```python
from build123d import *

# Parameters (mm, degrees)
SKETCH1_W           = 55
SKETCH1_H           = 35
SKETCH1_R           = 9.55
SKETCH1_R_2         = 1.5
BOSS_EXTRUDE3_DEPTH = 6
SKETCH4_W           = 55
SKETCH4_H           = 35
BOSS_EXTRUDE5_DEPTH = 2
SKETCH8_W           = 8.5
SKETCH8_H           = 35
BOSS_EXTRUDE6_DEPTH = 55
SKETCH9_R           = 2
CUT_EXTRUDE1_DEPTH  = 8.5
FILLET1_R           = 2


with BuildPart() as part:
    # Sketch1 → Boss-Extrude3 (new body)
    with BuildSketch(Plane.XY):
        with Locations((27.5, 17.5)):
            Rectangle(SKETCH1_W, SKETCH1_H)
        with Locations((35, 17.5)):
            Circle(SKETCH1_R, mode=Mode.SUBTRACT)
        with Locations((44.192388155, 26.692388155)):
            Circle(SKETCH1_R_2, mode=Mode.SUBTRACT)
        with Locations((44.192388155, 8.307611845)):
            Circle(SKETCH1_R_2, mode=Mode.SUBTRACT)
        with Locations((25.807611845, 8.307611845)):
            Circle(SKETCH1_R_2, mode=Mode.SUBTRACT)
        with Locations((25.807611845, 26.692388155)):
            Circle(SKETCH1_R_2, mode=Mode.SUBTRACT)
    extrude(amount=BOSS_EXTRUDE3_DEPTH)

    # Sketch4 → Boss-Extrude5 (add)
    with BuildSketch(Plane.XY.offset(6)):
        with Locations((27.5, 17.5)):
            Rectangle(SKETCH4_W, SKETCH4_H)
        with BuildLine():
            ThreePointArc((28.799419693, 26.47083501), (23.686291501, 28.813708499), (26.02916499, 23.700580307))
            ThreePointArc((26.02916499, 23.700580307), (26.263454109, 23.57743344), (26.255822455, 23.312861521))
            ThreePointArc((26.255822455, 23.312861521), (24.5, 17.5), (26.255822455, 11.687138479))
            ThreePointArc((26.255822455, 11.687138479), (26.263454109, 11.42256656), (26.02916499, 11.299419693))
            ThreePointArc((26.02916499, 11.299419693), (23.686291501, 6.186291501), (28.799419693, 8.52916499))
            ThreePointArc((28.799419693, 8.52916499), (28.92256656, 8.763454109), (29.187138479, 8.755822455))
            ThreePointArc((29.187138479, 8.755822455), (35, 7), (40.812861521, 8.755822455))
            ThreePointArc((40.812861521, 8.755822455), (41.07743344, 8.763454109), (41.200580307, 8.52916499))
            ThreePointArc((41.200580307, 8.52916499), (46.313708499, 6.186291501), (43.97083501, 11.299419693))
            ThreePointArc((43.97083501, 11.299419693), (43.736545891, 11.42256656), (43.744177545, 11.687138479))
            ThreePointArc((43.744177545, 11.687138479), (45.5, 17.5), (43.744177545, 23.312861521))
            ThreePointArc((43.744177545, 23.312861521), (43.736545891, 23.57743344), (43.97083501, 23.700580307))
            ThreePointArc((43.97083501, 23.700580307), (46.313708499, 28.813708499), (41.200580307, 26.47083501))
            ThreePointArc((41.200580307, 26.47083501), (41.07743344, 26.236545891), (40.812861521, 26.244177545))
            ThreePointArc((40.812861521, 26.244177545), (35, 28), (29.187138479, 26.244177545))
            ThreePointArc((29.187138479, 26.244177545), (28.92256656, 26.236545891), (28.799419693, 26.47083501))
        make_face(mode=Mode.SUBTRACT)
    extrude(amount=BOSS_EXTRUDE5_DEPTH)

    # Sketch8 → Boss-Extrude6 (add)
    with BuildSketch(Plane(origin=(0, 0, 0), x_dir=(-1, 0, 0), z_dir=(0, 0, -1))):
        with Locations((-4.25, 17.5)):
            Rectangle(SKETCH8_W, SKETCH8_H)
    extrude(amount=BOSS_EXTRUDE6_DEPTH)

    # Sketch9 → Cut-Extrude1 (cut)
    with BuildSketch(Plane.ZY):
        with Locations((-47, 27)):
            Circle(SKETCH9_R)
        with Locations((-47, 8)):
            Circle(SKETCH9_R)
        with Locations((-8.5, 27)):
            Circle(SKETCH9_R)
        with Locations((-8.5, 8)):
            Circle(SKETCH9_R)
        with Locations((-23.5, 17.5)):
            Circle(SKETCH9_R)
    extrude(amount=-CUT_EXTRUDE1_DEPTH, mode=Mode.SUBTRACT)

    # Fillet1
    fillet1_edges = [part.edges().sort_by_distance(p)[0] for p in [
        (8.5, 17.5, 0),
    ]]
    fillet(fillet1_edges, radius=FILLET1_R)


solid = part.part
```
Part model, mm, in its own coordinate system. A direction names the side the tool comes from. Coordinates: 2 decimals unless noted, no trailing zeros. Order: outer loops, then holes, each group sorted by start corner. A loop starts at its lowest first (then second) coordinate and runs counter-clockwise, first axis right, second up. Notation, with made-up numbers: (76.25, 72.5) - (102.25, 72.5) arc R23 cw to (102.25, 88.5) - close; hole circle Ø2 at (57, 65.5). An arc over 180 degrees is marked (long way). Return JSON: item names as keys, results as strings. Group by question number.
Item 1: Cut at C-C (x = 6.5). List the corners of the cut face in (y, z), plus the area to 3 significant figures.
Item 2: Cut at D-D (z = -40.5). List the corners of the cut face in (x, y), plus the area to 4 significant figures.
Item 3: Cut at A-A (x = 35). List the corners of the cut face in (y, z), plus the area to 3 significant figures.
Item 4: Which spindle directions (+Z, -Z, +X, -X, +Y, -Y) get a long thin tool onto all of the face, cutting with end or side? Do faces 4 (the face through (4.19, 19.483, -23.76)), 5 (the face through (27.5, 25.5, 0)), 6 (the face through (45.5, 17.4, 7)). Say none if no direction does.
Item 5: Pull direction Z, two halves, no side cores. Call faces 1 (the face through (7, 35, -14)), 2 (the face through (4.19, 9.352, -9.974)), 3 (the face through (39, 27, 6)): pulls with the +Z half, pulls with the -Z half, needs draft (parallel to the pull), parting line crosses it, or undercut.
Item 6: Cut at B-B (z = -23.5). List the corners of the cut face in (x, y).
Item 7: Pin check, flat tips, straight feed: pin 1 (2.5 mm diameter, centred on x = 44.19, y = 8.31, fed in from -Z); pin 2 (5.5 mm diameter, centred on x = 44.19, y = 26.69, fed in from -Z); pin 3 (5 mm diameter, centred on y = 31, z = -42.5, fed in from +X); pin 4 (3.5 mm diameter, centred on x = 25.81, y = 26.69, fed in from +Z). Stop position of each tip, or through.
Item 8: Drill centre lines: probe 1 along Y at (x, z) = (3, -47); probe 2 along Y at (x, z) = (3.5, -23.5); probe 3 along Y at (x, z) = (26.5, 2.5). Where is each one in solid material? Low to high. Write a range as from..to.
Check values:
{
 "1": {"outline": "(0, -55) - (35, -55) - (35, 8) - (0, 8) - close; hole circle Ø4 at (8, -47); hole circle Ø4 at (8, -8.5); hole circle Ø4 at (17.5, -23.5); hole circle Ø4 at (27, -47); hole circle Ø4 at (27, -8.5)", "area": "2,140 mm2"},
 "2": {"outline": "(0, 0) - (8.5, 0) - (8.5, 35) - (0, 35) - close", "area": "297.5 mm2"},
 "3": {"outline": "(0, 0) - (7.95, 0) - (7.95, 6) - (7, 6) - (7, 8) - (0, 8) - close; (27.05, 0) - (35, 0) - (35, 8) - (28, 8) - (28, 6) - (27.05, 6) - close", "area": "123 mm2"},
 "4": {"face 4": "+X, -X", "face 5": "-Z, +X, +Y, -Y", "face 6": "+Z"},
 "5": {"face 1": "needs draft", "face 2": "undercut", "face 3": "pulls with the +Z half"},
 "6": {"outline": "(0, 0) - (8.5, 0) - (8.5, 15.5) - (0, 15.5) - close; (0, 19.5) - (8.5, 19.5) - (8.5, 35) - (0, 35) - close"},
 "7": {"pin 1": "passes through", "pin 2": "stops at z = 0", "pin 3": "stops at x = 8.5", "pin 4": "stops at z = 6"},
 "8": {"probe 1": "y = 0..6, 10..25, 29..35", "probe 2": "y = 0..15.5, 19.5..35", "probe 3": "y = 0..6.98, 9.64..13.15, 21.85..25.36, 28.02..35"}
}
